```python
from build123d import *

# Parameters (mm, degrees)
MOTOR_PLATE_R       = 1.524
MOTOR_PLATE_R_2     = 5.969
BOSS_EXTRUDE1_DEPTH = 6.35


with BuildPart() as part:
    # Motor plate → Boss-Extrude1 (new body)
    with BuildSketch(Plane(origin=(0, 0, 0), x_dir=(0, 0, -1), z_dir=(1, 0, 0))):
        Polygon((-57.15, -19.853598803), (57.15, -19.853598803), (57.15, -26.203598803), (63.5, -26.203598803), (63.5, -19.853598803), (69.85, -19.853598803), (69.85, -14.318598824), (67.809000018, -14.318598824), (67.809000018, -11.418598782), (69.85, -11.418598782), (69.85, -5.883598803), (74.168, -5.883598803), (74.168, -11.418598782), (76.208999982, -11.418598782), (76.208999982, -14.318598824), (74.168, -14.318598824), (74.168, -19.853598803), (80.518, -19.853598803), (80.518, -26.203598803), (86.868, -26.203598803), (86.868, -19.853598803), (86.868, 19.853598803), (57.15, 19.853598803), (-57.15, 19.853598803), (-86.868, 19.853598803), (-86.868, -19.853598803), (-86.868, -26.203598803), (-80.518, -26.203598803), (-80.518, -19.853598803), (-74.168, -19.853598803), (-74.168, -14.318598824), (-76.208999982, -14.318598824), (-76.208999982, -11.418598782), (-74.168, -11.418598782), (-74.168, -5.883598803), (-69.85, -5.883598803), (-69.85, -11.418598782), (-67.809000018, -11.418598782), (-67.809000018, -14.318598824), (-69.85, -14.318598824), (-69.85, -19.853598803), (-63.5, -19.853598803), (-63.5, -26.203598803), (-57.15, -26.203598803), align=None)
        with Locations((-7.747, -14.856796409)):
            Circle(MOTOR_PLATE_R, mode=Mode.SUBTRACT)
        with Locations((0, -8.550598803)):
            Circle(MOTOR_PLATE_R_2, mode=Mode.SUBTRACT)
        with Locations((7.747, -14.856796409)):
            Circle(MOTOR_PLATE_R, mode=Mode.SUBTRACT)
        with Locations((-15.494, -1.438598803)):
            Circle(MOTOR_PLATE_R, mode=Mode.SUBTRACT)
        with Locations((-7.747, 11.979598803)):
            Circle(MOTOR_PLATE_R, mode=Mode.SUBTRACT)
        with Locations((15.494, -1.438598803)):
            Circle(MOTOR_PLATE_R, mode=Mode.SUBTRACT)
        with Locations((7.747, 11.979598803)):
            Circle(MOTOR_PLATE_R, mode=Mode.SUBTRACT)
    extrude(amount=BOSS_EXTRUDE1_DEPTH)


solid = part.part
```
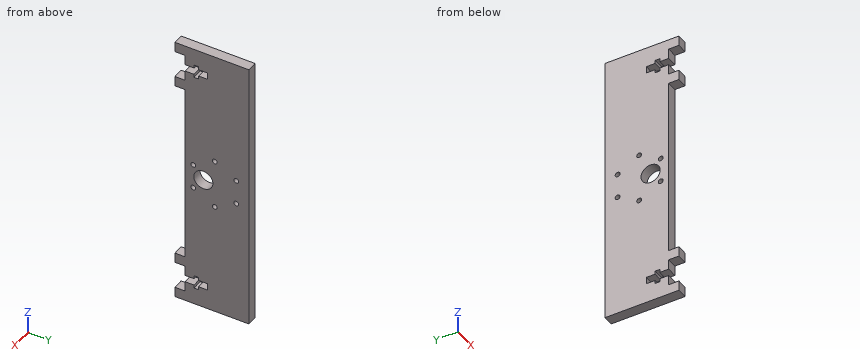
Verification items for the finished model (mm, model axes). Coordinates: 2 decimals unless noted, no trailing zeros. Loops run counter-clockwise (first coordinate to the right, second up) from the corner with the lowest first, then second, coordinate; pieces in that order, holes last. Notation, with made-up numbers: (-19, -15) -> (7, -15) arc R13 ccw to (7, 10) -> close; hole circle Ø4 at (68.5, -37). An arc over 180 degrees is marked (long way). Put each result on its own line as item: value.
1. Section check B-B, the plane z = 37. Record the boundary of the cut face in (x, y).
Result set:
outline: (0, -19.85) -> (6.35, -19.85) -> (6.35, 19.85) -> (0, 19.85) -> close
2. Gauge pin test, flat end, axial feed: P1, Ø3, axis at x = 3, z = -36.5, coming from the -Y side. Record the tip position at first contact, or that the pin passes through.
Result set:
P1: stops at y = -19.85
3. Section check A-A, the plane z = 0. Record the boundary of the cut face in (x, y), then the cut area to 3 significant figures.
Result set:
outline: (0, -19.85) -> (6.35, -19.85) -> (6.35, -14.52) -> (0, -14.52) -> close; (0, -2.58) -> (6.35, -2.58) -> (6.35, 19.85) -> (0, 19.85) -> close
area: 176 mm^2
4. Thickness scan on line 1 (Z direction, x = 3.25, y = -21.5); line 2 (Z direction, x = 2, y = -2); line 3 (Y direction, x = 3.75, z = 0). Record the ranges inside material, lowest first.
Result set:
line 1: z = -86.87 to -80.52, -63.5 to -57.15, 57.15 to 63.5, 80.52 to 86.87
line 2: z = -86.87 to -16.91, -14.08 to 14.08, 16.91 to 86.87
line 3: y = -19.85 to -14.52, -2.58 to 19.85
5. Section check C-C, the plane x = 4.25. Give the number of separate pieces and of enclosed holes in the cut face, then the cut area to 3 significant figures.
Result set:
separate pieces: 1
enclosed holes: 7
area: 6,760 mm^2
